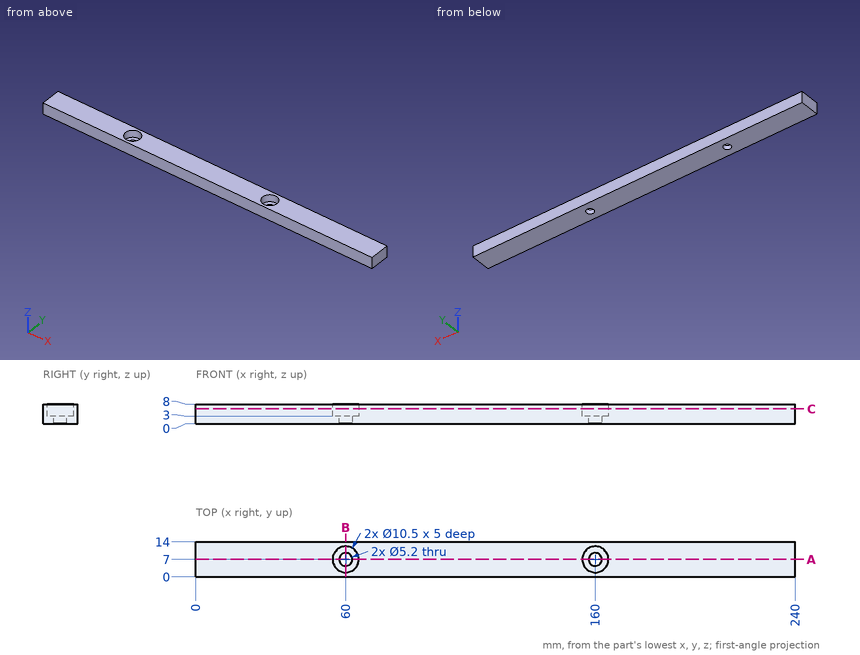
Geometry check sheet. Reference: drawing and pictorial views, mm from the part's lowest x, y, z. Coordinates: 2 decimals unless noted, no trailing zeros. Loops run counter-clockwise (first coordinate to the right, second up) from the corner with the lowest first, then second, coordinate; pieces in that order, holes last.
1) Gauge pin test, flat ends, axial feed: pin 1 (4.5 mm diameter, centred on x = 60, y = 7, fed in from +Z); pin 2 (6.5 mm diameter, centred on x = 60, y = 7, fed in from +Z). Record the tip position at first contact, or that the pin passes through.
2) Sectioned sample at C-C (z = 6). Record the boundary of the cut face in (x, y), and give its area (3 significant figures).
3) Material ranges on probe 1 along Y at (x, z) = (160, 1.8); probe 2 along X at (y, z) = (8.25, 5.75); probe 3 along X at (y, z) = (9, 1.75), recorded low to high.
4) Sectioned sample at B-B (x = 60). Record the boundary of the cut face in (y, z), and give its area (3 significant figures).
5) Sectioned sample at A-A (y = 7). Record the boundary of the cut face in (x, z).
Check sheet entries:
1. pin 1: passes through
1. pin 2: stops at z = 3
2. outline: (0, 0) - (240, 0) - (240, 14) - (0, 14) - close; hole circle Ø10.5 at (60, 7); hole circle Ø10.5 at (160, 7)
2. area: 3,190 mm2
3. probe 1: y = 0 to 4.4, 9.6 to 14
3. probe 2: x = 0 to 54.9, 65.1 to 154.9, 165.1 to 240
3. probe 3: x = 0 to 58.34, 61.66 to 158.34, 161.66 to 240
4. outline: (0, 0) - (4.4, 0) - (4.4, 3) - (1.75, 3) - (1.75, 8) - (0, 8) - close; (9.6, 0) - (14, 0) - (14, 8) - (12.25, 8) - (12.25, 3) - (9.6, 3) - close
4. area: 43.9 mm2
5. outline: (0, 0) - (57.4, 0) - (57.4, 3) - (54.75, 3) - (54.75, 8) - (0, 8) - close; (62.6, 0) - (157.4, 0) - (157.4, 3) - (154.75, 3) - (154.75, 8) - (65.25, 8) - (65.25, 3) - (62.6, 3) - close; (162.6, 0) - (240, 0) - (240, 8) - (165.25, 8) - (165.25, 3) - (162.6, 3) - close
